from build123d import *

# Parameters (mm, degrees)
PAD_DEPTH       = 10
CHAMFER_SIZE    = 0.5
CHAMFER001_SIZE = 0.5


with BuildPart() as part:
    # Sketch → Pad (new body)
    with BuildSketch(Plane.XZ):
        with BuildLine():
            ThreePointArc((-1.5, 3.162278), (0, -3.5), (1.5, 3.162278))
            Line((1.5, 3.162278), (2.5, 4.330127))
            ThreePointArc((5, 2.7e-05), (4.33012, 2.500012), (2.5, 4.330127))
            Line((5, -3.669873), (5, 2.7e-05))
            Line((8.5, -3.669873), (5, -3.669873))
            Line((8.5, -5.669873), (8.5, -3.669873))
            Line((-8.5, -5.669873), (8.5, -5.669873))
            Line((-8.5, -3.669873), (-8.5, -5.669873))
            Line((-5, -3.669873), (-8.5, -3.669873))
            Line((-5, 2.7e-05), (-5, -3.669873))
            ThreePointArc((-2.5, 4.330127), (-4.33012, 2.500012), (-5, 2.7e-05))
            Line((-2.5, 4.330127), (-1.5, 3.162278))
        make_face()
    extrude(amount=PAD_DEPTH)

    # Chamfer
    chamfer_edges = [part.edges().sort_by_distance(p)[0] for p in [
        (-2.5, -5, 4.330127),
    ]]
    chamfer(chamfer_edges, length=CHAMFER_SIZE)

    # Chamfer001
    chamfer001_edges = [part.edges().sort_by_distance(p)[0] for p in [
        (2.5, -5, 4.330127),
    ]]
    chamfer(chamfer001_edges, length=CHAMFER001_SIZE)


solid = part.part
CAD build for the part. Positions are in the model's coordinates, mm. A direction names the side the tool comes from. Give positions to 0.01 mm unless a question says otherwise; leave off trailing zeros. Loops run counter-clockwise (first coordinate to the right, second up) from the corner with the lowest first, then second, coordinate; pieces in that order, holes last. Notation, with made-up numbers: M 72.25,83.5 L 85.25,83.5 A7 cw 85.25,94.5 Z; hole C 65.5,-33.75 d8. An arc over 180 degrees is marked long. One line per question, with ' | ' between items. Start each with the question number.
1. Two-plate mould, pull along X, no slides. Class faces 1 (the face through (-4.434, -4.93, 2.31)), 2 (the face through (-0.1, -4.9, -3.5)), 3 (the face through (0, -10, -4)): pulls with the +X half, pulls with the -X half, needs draft (parallel to the pull), parting line crosses it, or undercut.
2. Saw through at C-C on y = -7.25. Give the cut face in (x, z), plus the area to 3 significant figures.
3. Saw through at B-B on x = 3.25. Give the cut face in (y, z), plus the area to 3 significant figures.
4. Flat gauge pins, fed straight in: pin 1 (3 mm diameter, centred on x = 6, y = -5, fed in from +Z); pin 2 (1.1 mm diameter, centred on y = -4.5, z = -1.5, fed in from -X); pin 3 (4 mm diameter, centred on y = -4.5, z = -1, fed in from +X). Where does each tip first touch, or does it go through?
5. Saw through at D-D on x = -7. Give the cut face in (y, z), plus the area to 3 significant figures.
6. 3-axis set-ups, long thin cutter, end or side, ignore diameter. For faces 4 (the face through (8.5, -5, -5)), 5 (the face through (-5, -5, -2)), 6 (the face through (5, -5, -2)): which of +Z, -Z, +X, -X, +Y, -Y reach the whole face in a straight line?
7. Saw through at A-A on z = 0.25. Give the cut face in (x, y).
8. Probe L1, parallel to X at y = -7, z = 0; L2, parallel to X at y = -3, z = -2; L3, parallel to Z at x = -2, y = -2. List the from-to ranges inside material, lowest first. Write a range as from..to.
Result sheet:
1) face 1: pulls with the -X half | face 2: undercut | face 3: needs draft
2) outline: M -8.5,-5.67 L 8.5,-5.67 L 8.5,-3.67 L 5,-3.67 L 5,0 A5 ccw 2.92,4.06 L 2.17,3.95 L 1.5,3.16 A3.5 cw long -1.5,3.16 L -2.17,3.95 L -2.92,4.06 A5 ccw -5,0 L -5,-3.67 L -8.5,-3.67 Z | area: 65.0 mm^2
3) outline: M -10,-5.67 L 0,-5.67 L 0,-1.3 L -10,-1.3 Z; M -10,1.3 L 0,1.3 L 0,3.8 L -10,3.8 Z | area: 68.7 mm^2
4) pin 1: stops at z = 2.18 | pin 2: stops at x = -5 | pin 3: stops at x = 5
5) outline: M -10,-5.67 L 0,-5.67 L 0,-3.67 L -10,-3.67 Z | area: 20.0 mm^2
6) face 4: +Z, -Z, +X, +Y, -Y | face 5: +Z, -X, +Y, -Y | face 6: +Z, +X, +Y, -Y
7) outline: M -4.99,-10 L -3.49,-10 L -3.49,0 L -4.99,0 Z; M 3.49,-10 L 4.99,-10 L 4.99,0 L 3.49,0 Z
8) L1: x = -5..-3.5, 3.5..5 | L2: x = -5..-2.87, 2.87..5 | L3: z = -5.67..-2.87, 2.87..3.75
